from build123d import *

# Parameters (mm, degrees)
BOSS_EXTRUDE1_DEPTH = 120
SKETCH2_R           = 12.5
CUT_EXTRUDE1_DEPTH  = 80


with BuildPart() as part:
    # Sketch1 → Boss-Extrude1 (new body)
    with BuildSketch(Plane.XY):
        with BuildLine():
            Line((-89.876617225, -13.45998777), (-89.876617225, 13.45998777))
            add(Edge.make_bspline(
                [(89.876617225, 13.45998777), (0, 74.633199683), (-89.876617225, 13.45998777)],
                knots=[3.580195105, 3.580195105, 3.580195105, 5.844582856, 5.844582856, 5.844582856], degree=2, weights=[1, 0.424674615, 1]))
            Line((89.876617225, 13.45998777), (89.876617225, -13.45998777))
            add(Edge.make_bspline(
                [(-89.876617225, -13.45998777), (0, -74.633199683), (89.876617225, -13.45998777)],
                knots=[0.438602452, 0.438602452, 0.438602452, 2.702990202, 2.702990202, 2.702990202], degree=2, weights=[1, 0.424674615, 1]))
        make_face()
    extrude(amount=BOSS_EXTRUDE1_DEPTH)

    # Sketch2 → Cut-Extrude1 (cut)
    with BuildSketch(Plane.XY.offset(120)):
        with Locations((-67.358364495, 0)):
            Circle(SKETCH2_R)
        with Locations(Location((67.358364495, 0, 0), (0, 0, 180))):
            Circle(SKETCH2_R)
    extrude(amount=-CUT_EXTRUDE1_DEPTH, mode=Mode.SUBTRACT)


solid = part.part
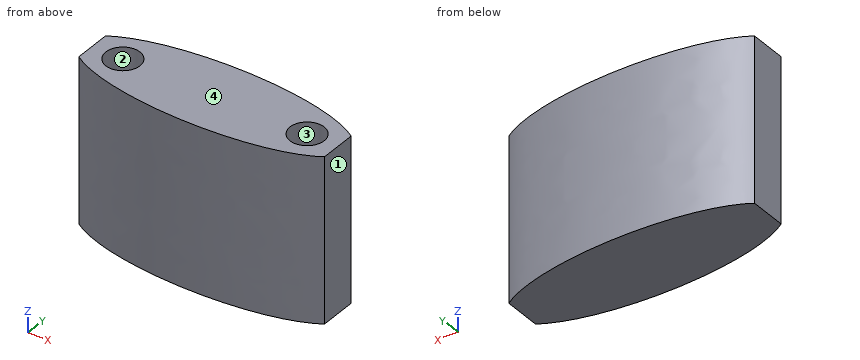
Check sheet for the modelled part. Datum: model origin and axes. Units: mm. Face numbers are marked on the shaded views. A direction names the side the tool comes from. Round coordinates to 2 decimals unless told otherwise and drop trailing zeros. Loops run counter-clockwise (first coordinate to the right, second up) from the corner with the lowest first, then second, coordinate; pieces in that order, holes last.
1. Gauge pin test, flat ends, axial feed: pin 1 Ø4 at (x, z) = (-57.5, 13.5) entering from -Y; pin 2 Ø12.5 at (x, y) = (67.5, -3) entering from +Z; pin 3 Ø2 at (y, z) = (17.5, 49) entering from -X. Record the tip position at first contact, or that the pin passes through.
2. Scan lines: probe 1 along X at (y, z) = (2.5, 51.5); probe 2 along Z at (x, y) = (-60, -2); probe 3 along Y at (x, z) = (-61, 69). Record each from-to range of solid material in increasing order.
3. Sectioned sample at A-A on y = 0. Record the boundary of the cut face in (x, z).
4. Sectioned sample at B-B on z = 104. Give the number of separate pieces and of enclosed holes in the cut face, and give its area (3 significant figures).
5. Mould release check, pull along Y, two halves, no side actions. Record for the marked faces 3 and 4: released by +Y, released by -Y, zero draft, split by the parting line, or undercut.
6. Sectioned sample at C-C on y = 10.5. Record the boundary of the cut face in (x, z).
7. Set-up check for the marked faces 1 and 2: record each of +Z, -Z, +X, -X, +Y, -Y from which the full face is reachable in a straight line by a thin tool's end or side.
Recorded:
1. pin 1: stops at y = -26.28
1. pin 2: stops at z = 40
1. pin 3: stops at x = -84.76
2. probe 1: x = -89.88 to -79.61, -55.11 to 55.11, 79.61 to 89.88
2. probe 2: z = 0 to 40
2. probe 3: y = -25.01 to -10.76, 10.76 to 25.01
3. outline: (-89.88, 0) - (89.88, 0) - (89.88, 120) - (79.86, 120) - (79.86, 40) - (54.86, 40) - (54.86, 120) - (-54.86, 120) - (-54.86, 40) - (-79.86, 40) - (-79.86, 120) - (-89.88, 120) - close
4. separate pieces: 1
4. enclosed holes: 2
4. area: 8,560 mm2
5. face 3: undercut
5. face 4: zero draft
6. outline: (-89.88, 0) - (89.88, 0) - (89.88, 120) - (74.14, 120) - (74.14, 40) - (60.58, 40) - (60.58, 120) - (-60.58, 120) - (-60.58, 40) - (-74.14, 40) - (-74.14, 120) - (-89.88, 120) - close
7. face 1: +Z, -Z, +X, +Y, -Y
7. face 2: +Z
